The figure shows three views and two pictorial views of one solid part (mm, origin at its lowest corner). Answer the questions. A direction names the side the tool comes from. Coordinates: 2 decimals unless noted, no trailing zeros. Write each loop counter-clockwise with the first axis right and the second up, starting at its lowest first coordinate (ties: lowest second). Pieces come first, ordered by that corner, then holes. Notation, with made-up numbers: M 38.25,3.25 L 68.25,3.25 A15 ccw 68.25,31.25 Z; hole C 15.25,-9 d1. An arc over 180 degrees is marked long. Answer as CSV lines item,"result".
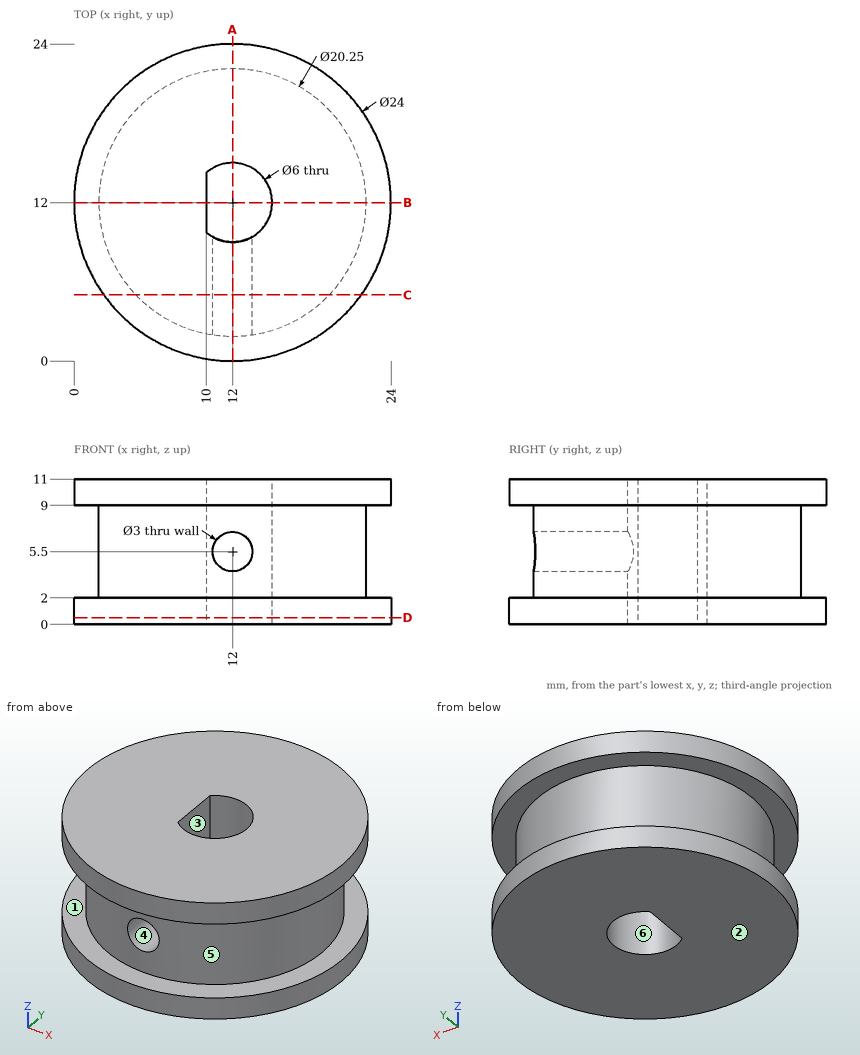
Q1. Find section D-D (z = 0.5). Give the vertices of the cut face in (x, y), and give its area (3 significant figures).
Output:
outline,"C 12,12 d24; hole M 10,9.76 A3 ccw long 10,14.24 Z"
area,"427 mm2"
Q2. Find section C-C (y = 5). Give the vertices of the cut face in (x, z).
Output:
outline,"M 2.25,0 L 21.75,0 L 21.75,2 L 19.32,2 L 19.32,9 L 21.75,9 L 21.75,11 L 2.25,11 L 2.25,9 L 4.68,9 L 4.68,2 L 2.25,2 Z; hole C 12,5.5 d3"
Q3. Straight lines are drawn through the part: line 1 (Z direction, x = 6.75, y = 21.5); line 2 (Z direction, x = 12, y = 7); line 3 (Y direction, x = 12, z = 8) (3 decimals). For each, find the intervals that lie inside material, in ascending order.
Output:
line 1,"0 to 2, 9 to 11"
line 2,"0 to 4, 7 to 11"
line 3,"1.875 to 9, 15 to 22.125"
Q4. For the marked faces 1 and 2, determine the directions among +Z, -Z, +X, -X, +Y, -Y from which every point of the face is accessible in a straight line to the end or side of a thin tool.
Output:
face 1,"none"
face 2,"-Z, +X, -X, +Y, -Y"
Q5. Find section A-A (x = 12). Give the vertices of the cut face in (y, z) (3 decimals).
Output:
outline,"M 0,0 L 9,0 L 9,4 L 1.875,4 L 1.875,2 L 0,2 Z; M 0,9 L 1.875,9 L 1.875,7 L 9,7 L 9,11 L 0,11 Z; M 15,0 L 24,0 L 24,2 L 22.125,2 L 22.125,9 L 24,9 L 24,11 L 15,11 Z"
Q6. Flat-ended cylindrical pins translate along their axes: pin 1 Ø3.5 at (x, z) = (12, 5.5) entering from +Y (3 decimals); pin 2 Ø4 at (x, z) = (3, 6) entering from +Y; pin 3 Ø1.3 at (y, z) = (12.5, 5) entering from +X (3 decimals). Find the tip coordinate at first contact, or state that the pin passes through.
Output:
pin 1,"y = 22.125"
pin 2,"y = 19.32"
pin 3,"x = 22.125"
Q7. The mould has two halves that part along Y. Classify the marked faces 3, 4, 5 and 6: pulls with the +Y half, pulls with the -Y half, needs draft (parallel to the pull), parting line crosses it, or undercut.
Output:
face 3,"undercut"
face 4,"needs draft"
face 5,"parting line crosses it"
face 6,"undercut"
Q8. Find section B-B (y = 12). Give the vertices of the cut face in (x, z) (3 decimals), and give its area (3 significant figures).
Output:
outline,"M 0,0 L 10,0 L 10,11 L 0,11 L 0,9 L 1.875,9 L 1.875,2 L 0,2 Z; M 15,0 L 24,0 L 24,2 L 22.125,2 L 22.125,9 L 24,9 L 24,11 L 15,11 Z"
area,"183 mm2"
